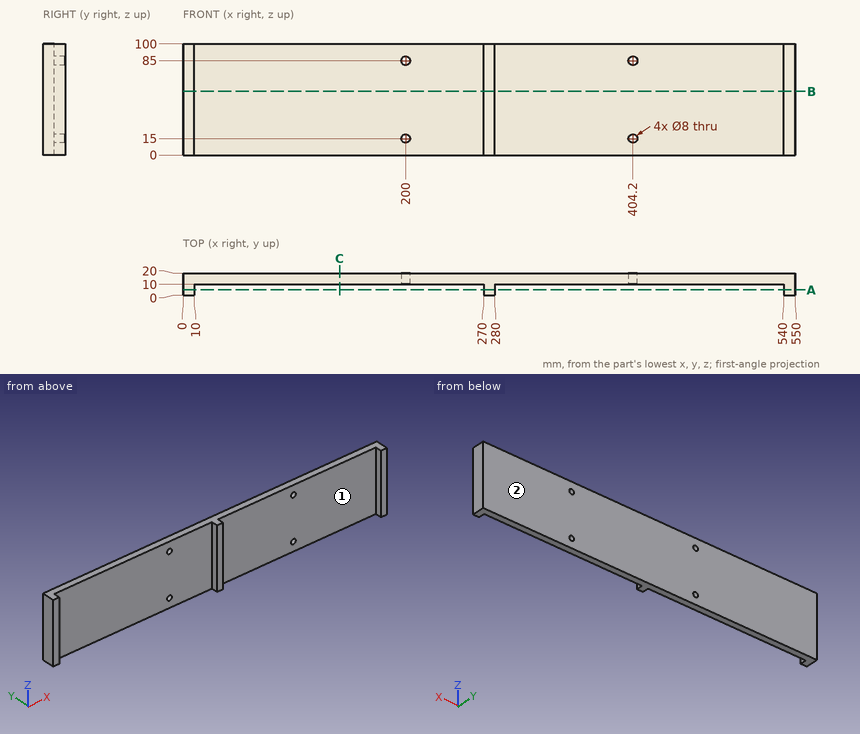
Can you work these out from the drawing? Everything is in mm from the part's minimum corner. Round coordinates to 2 decimals unless told otherwise and drop trailing zeros. Loops run counter-clockwise (first coordinate to the right, second up) from the corner with the lowest first, then second, coordinate; pieces in that order, holes last. Notation, with made-up numbers: M -36.75,41.5 L -1.75,41.5 A11 cw -1.75,54.5 Z; hole C 67.5,-30 d5. An arc over 180 degrees is marked long. Write item = value, one per line.
1. I want a section at A-A, the plane y = 5. Write out the boundary of the cut face in (x, z), and give its area (3 significant figures).
Results below:
outline = M 0,0 L 10,0 L 10,100 L 0,100 Z; M 270,0 L 280,0 L 280,100 L 270,100 Z; M 540,0 L 550,0 L 550,100 L 540,100 Z
area = 3,000 mm²
2. Will this pin go through, and if not, where does the flat tip stop? P1, Ø13, axis at x = 200, z = 85, coming from the -Y side.
Results below:
P1 = 10
3. I need wall thicknesses on probe 1 along X at (y, z) = (12.75, 15); probe 2 along Z at (x, y) = (404.2, 16.25); probe 3 along X at (y, z) = (3.75, 41). Which ranges of each line are inside material? Lowest first, please.
Results below:
probe_1 = 0 to 196, 204 to 400.2, 408.2 to 550
probe_2 = 0 to 11, 19 to 81, 89 to 100
probe_3 = 0 to 10, 270 to 280, 540 to 550
4. Thinking about a two-plate mould opening in X: for the marked faces 1 and 2, which applies, +X half, -X half, draft (parallel to the pull), parting line (faces both ways), or undercut?
Results below:
face_1 = undercut
face_2 = draft
5. I want a section at C-C, the plane x = 140.5. Write out the boundary of the cut face in (y, z).
Results below:
outline = M 10,0 L 20,0 L 20,100 L 10,100 Z
6. I want a section at B-B, the plane z = 57.5. Write out the boundary of the cut face in (x, y).
Results below:
outline = M 0,0 L 10,0 L 10,10 L 270,10 L 270,0 L 280,0 L 280,10 L 540,10 L 540,0 L 550,0 L 550,20 L 0,20 Z
